Model file for the job. Use its own axes, mm. Face numbers are marked on the shaded views. A direction names the side the tool comes from. Give positions to 0.01 mm unless a question says otherwise; leave off trailing zeros. Write each loop counter-clockwise with the first axis right and the second up, starting at its lowest first coordinate (ties: lowest second). Pieces come first, ordered by that corner, then holes. Notation, with made-up numbers: (0, 85) - (56, 85) arc R35 cw to (56, 120) - close; hole circle Ø3 at (79.25, 23). An arc over 180 degrees is marked (long way). One line per item, written item: value. Start each with the question number.
(1) Drop flat-ended pins along their axis: P1, Ø6, axis at y = 5.5, z = -4.5, coming from the -X side; P2, Ø2, axis at y = 13, z = -9.5, coming from the -X side; P3, Ø3, axis at y = 13.5, z = 5, coming from the +X side; P4, Ø2, axis at y = 6.5, z = -9.5, coming from the -X side (3 decimals). Give the stop position or say it passes through.
(2) 3-axis set-ups, long thin cutter, end or side, ignore diameter. For the marked faces 1, 2, 3 and 4: which of +Z, -Z, +X, -X, +Y, -Y reach the whole face in a straight line?
(3) Probe L1, parallel to Z at x = -2, y = 5.25; L2, parallel to Y at x = 4, z = -6. List the from-to ranges inside material, lowest first.
(4) Cut at B-B, the plane z = 0. List the corners of the cut face in (x, y) (3 decimals), and give its area (3 significant figures).
(5) Cut at C-C, the plane x = 0. List the corners of the cut face in (y, z) (3 decimals), and give its area (3 significant figures).
(6) Cut at A-A, the plane y = 9.75. List the corners of the cut face in (x, z), and give its area (3 significant figures).
from build123d import *

# Parameters (mm, degrees)
SKETCH1_W           = 14.4
SKETCH1_H           = 14.4
BOSS_EXTRUDE1_DEPTH = 19.7
SKETCH3_R           = 2.375
BOSS_EXTRUDE2_DEPTH = 12
SKETCH4_R           = 2.375
BOSS_EXTRUDE3_DEPTH = 12
CHAMFER1_SIZE       = 0.3
CHAMFER2_SIZE       = 0.5


with BuildPart() as part:
    # Sketch1 → Boss-Extrude1 (new body)
    with BuildSketch(Plane(origin=(0, 0, 0), x_dir=(1, 0, 0), z_dir=(0, 1, 0))):
        Rectangle(SKETCH1_W, SKETCH1_H)
    extrude(amount=BOSS_EXTRUDE1_DEPTH)

    # Sketch2 → Cut-Revolve1 (revolve, cut)
    with BuildSketch(Plane.XY, mode=Mode.PRIVATE) as cut_revolve1_sk:
        Polygon((-6.95, 19.7), (-16.09, 19.7), (-16.09, 0), (-6.95, 0), (-13.55, 3.810511777), (-13.55, 15.889488223), align=None)
    revolve(cut_revolve1_sk.sketch.rotate(Axis((0, 20.685, 0), (0, -1, 0)), 270), axis=Axis((0, 20.685, 0), (0, -1, 0)), mode=Mode.SUBTRACT)

    # Sketch3 → Boss-Extrude2 (add, symmetric)
    with BuildSketch(Plane.XY):
        with Locations(Location((0, 6.7, 0), (0, 0, 180))):
            Circle(SKETCH3_R)
    extrude(amount=BOSS_EXTRUDE2_DEPTH, both=True)

    # Sketch4 → Boss-Extrude3 (add, symmetric)
    with BuildSketch(Plane(origin=(0, 0, 0), x_dir=(0, 0, -1), z_dir=(1, 0, 0))):
        with Locations((0, 13)):
            Circle(SKETCH4_R)
    extrude(amount=BOSS_EXTRUDE3_DEPTH, both=True)

    # Chamfer1
    chamfer1_edges = [part.edges().sort_by_distance(p)[0] for p in [
        (2.375, 6.7, -12),
        (2.375, 6.7, 12),
        (-12, 13, 2.375),
        (12, 13, 2.375),
    ]]
    chamfer(chamfer1_edges, length=CHAMFER1_SIZE)

    # Chamfer2
    chamfer2_edges = [part.edges().sort_by_distance(p)[0] for p in [
        (7.2, 9.85, 7.2),
        (7.2, 9.85, -7.2),
        (-7.2, 9.85, 7.2),
        (-7.2, 9.85, -7.2),
    ]]
    chamfer(chamfer2_edges, length=CHAMFER2_SIZE)


solid = part.part
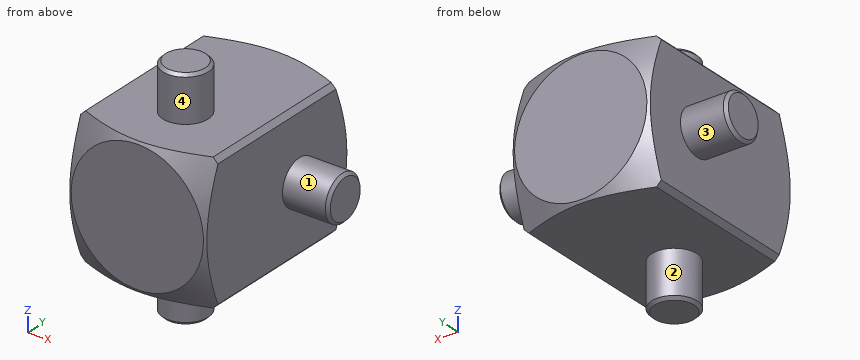
Answers follow:
1. P1: stops at x = -7.2
1. P2: passes through
1. P3: stops at x = 7.2
1. P4: stops at x = -2.375
2. face 1: +X
2. face 2: -Z
2. face 3: -X
2. face 4: +Z
3. L1: z = -7.2 to 7.2
3. L2: y = 0.15 to 19.55
4. outline: (-12, 10.925) - (-11.7, 10.625) - (-7.2, 10.625) - (-7.2, 0.144) - (-6.95, 0) - (6.95, 0) - (7.2, 0.144) - (7.2, 10.625) - (11.7, 10.625) - (12, 10.925) - (12, 15.075) - (11.7, 15.375) - (7.2, 15.375) - (7.2, 19.556) - (6.95, 19.7) - (-6.95, 19.7) - (-7.2, 19.556) - (-7.2, 15.375) - (-11.7, 15.375) - (-12, 15.075) - close
4. area: 329 mm²
5. outline: (0, -6.95) - (0.144, -7.2) - (4.325, -7.2) - (4.325, -11.7) - (4.625, -12) - (8.775, -12) - (9.075, -11.7) - (9.075, -7.2) - (19.556, -7.2) - (19.7, -6.95) - (19.7, 6.95) - (19.556, 7.2) - (9.075, 7.2) - (9.075, 11.7) - (8.775, 12) - (4.625, 12) - (4.325, 11.7) - (4.325, 7.2) - (0.144, 7.2) - (0, 6.95) - close
5. area: 329 mm²
6. outline: (-7.2, -6.7) - (-6.7, -7.2) - (6.7, -7.2) - (7.2, -6.7) - (7.2, 6.7) - (6.7, 7.2) - (-6.7, 7.2) - (-7.2, 6.7) - close
6. area: 207 mm²
